```python
from build123d import *

# Parameters (mm, degrees)
F0_W     = 254
F0_H     = 101.6
F1_DEPTH = 12.7
F2_R     = 10.16
F3_DEPTH = 25.4
F4_R     = 6.35


with BuildPart() as f1:
    # F0 (on Front) → F1 (new body)
    with BuildSketch(Plane.XZ):
        with Locations((127, 50.8)):
            Rectangle(F0_W, F0_H)
    extrude(amount=F1_DEPTH)

    # F2 (on face) → F3 (cut)
    with BuildSketch(Plane.XZ.offset(12.7)):
        with Locations((50.8, 50.8)):
            Circle(F2_R)
        with Locations((203.2, 50.8)):
            Circle(F2_R)
    extrude(amount=-F3_DEPTH, mode=Mode.SUBTRACT)

    # F4
    f4_edges = [f1.edges().sort_by_distance(p)[0] for p in [
        (0, -6.35, 101.6),
        (254, -6.35, 101.6),
        (254, -6.35, 0),
        (0, -6.35, 0),
    ]]
    fillet(f4_edges, radius=F4_R)


solid = f1.part
```
Work out the finished part from the listing and answer in its coordinate system (mm). Round coordinates to 2 decimals unless told otherwise and drop trailing zeros. Write each loop counter-clockwise with the first axis right and the second up, starting at its lowest first coordinate (ties: lowest second). Pieces come first, ordered by that corner, then holes. Notation, with made-up numbers: (45.5, 68) -> (93.5, 68) arc R13 ccw to (93.5, 77) -> close; hole circle Ø5 at (28.25, 58). An arc over 180 degrees is marked (long way). Write each question's results on one line, items separated by ' | '.
1) A flat-ended cylindrical pin translates along its axis: pin 1 (12 mm diameter, centred on x = 203.2, z = 50.8, fed in from +Y). Find the tip coordinate at first contact, or state that the pin passes through.
Findings:
pin 1: passes through
2) For a pull along X with two mould halves and no side action, classify faces 1 (the cylindrical face through (252.09, -6.44, 99.79)), 2 (the cylindrical face through (49.477, -6.439, 60.874)), 3 (the flat face through (125, -6, 101.6)) as +X half, -X half, draft (parallel to the pull), parting line (faces both ways), or undercut.
Findings:
face 1: +X half | face 2: undercut | face 3: draft
3) The part is cut by section A-A (x = 50.8). Write down the section's boundary in (y, z).
Findings:
outline: (-12.7, 0) -> (0, 0) -> (0, 40.64) -> (-12.7, 40.64) -> close; (-12.7, 60.96) -> (0, 60.96) -> (0, 101.6) -> (-12.7, 101.6) -> close
4) The part is cut by section C-C (y = -10). Write down the section's boundary in (x, z), and give its area (3 significant figures).
Findings:
outline: (0, 6.35) arc R6.35 ccw to (6.35, 0) -> (247.65, 0) arc R6.35 ccw to (254, 6.35) -> (254, 95.25) arc R6.35 ccw to (247.65, 101.6) -> (6.35, 101.6) arc R6.35 ccw to (0, 95.25) -> close; hole circle Ø20.32 at (50.8, 50.8); hole circle Ø20.32 at (203.2, 50.8) | area: 25,100 mm²
5) Consider line 1 along X through (y, z) = (-3.75, 56.5); line 2 along Z through (x, y) = (203.2, -8.5); line 3 along X through (y, z) = (-9.5, 55). Determine where each line is inside the solid, lowest interval first. Write a range as [from, to].
Findings:
line 1: x = [0, 42.39], [59.21, 194.79], [211.61, 254] | line 2: z = [0, 40.64], [60.96, 101.6] | line 3: x = [0, 41.55], [60.05, 193.95], [212.45, 254]
6) The part is cut by section B-B (z = 50.8). Write down the section's boundary in (x, y), and give its area (3 significant figures).
Findings:
outline: (0, -12.7) -> (40.64, -12.7) -> (40.64, 0) -> (0, 0) -> close; (60.96, -12.7) -> (193.04, -12.7) -> (193.04, 0) -> (60.96, 0) -> close; (213.36, -12.7) -> (254, -12.7) -> (254, 0) -> (213.36, 0) -> close | area: 2,710 mm²
